from build123d import *

# Parameters (mm, degrees)
SKETCH_1_R      = 1
EXTRUDE_1_DEPTH = 1


with BuildPart() as part:
    # 草图1 → 凸台-拉伸1 (new body)
    with BuildSketch(Plane.XY):
        with BuildLine():
            Line((-1.5, 0), (-1.5, 16))
            ThreePointArc((-1.5, 16), (0, 17.5), (1.5, 16))
            Line((1.5, 16), (1.5, 0))
            ThreePointArc((1.5, 0), (0, -1.5), (-1.5, 0))
        make_face()
        with Locations((0, 16)):
            Circle(SKETCH_1_R, mode=Mode.SUBTRACT)
        with Locations((0, 8)):
            Circle(SKETCH_1_R, mode=Mode.SUBTRACT)
        with Locations((0, 12)):
            Circle(SKETCH_1_R, mode=Mode.SUBTRACT)
        Circle(SKETCH_1_R, mode=Mode.SUBTRACT)
        with Locations((0, 4)):
            Circle(SKETCH_1_R, mode=Mode.SUBTRACT)
    extrude(amount=EXTRUDE_1_DEPTH)


solid = part.part
The listing builds one solid part. Answer for the finished solid, in the listing's coordinates (mm). Round coordinates to 2 decimals unless told otherwise and drop trailing zeros. Loops run counter-clockwise (first coordinate to the right, second up) from the corner with the lowest first, then second, coordinate; pieces in that order, holes last. Notation, with made-up numbers: M -9.5,2.5 L 40.5,2.5 A16 ccw 40.5,19.5 Z; hole C 44.25,31.5 d4. An arc over 180 degrees is marked long. Return JSON: item names as keys, results as strings.
Q1. The mould has two halves that part along X. Classify faces 1 (the face through (-0.13, 4.99, 0.49)), 2 (the face through (1.5, 8.1, 0.5)), 3 (the face through (0, 17.5, 0.5)), 4 (the face through (-1.3, 8.1, 1)): released by +X, released by -X, zero draft, split by the parting line, or undercut.
Results list:
{"face 1": "undercut", "face 2": "released by +X", "face 3": "split by the parting line", "face 4": "zero draft"}
Q2. Find section B-B, the plane z = 0.3. Determine the outline of the cut face in (x, y).
Results list:
{"outline": "M -1.5,0 A1.5 ccw 1.5,0 L 1.5,16 A1.5 ccw -1.5,16 Z; hole C 0,0 d2; hole C 0,4 d2; hole C 0,8 d2; hole C 0,12 d2; hole C 0,16 d2"}
Q3. Find section A-A, the plane y = 8. Determine the outline of the cut face in (x, z).
Results list:
{"outline": "M -1.5,0 L -1,0 L -1,1 L -1.5,1 Z; M 1,0 L 1.5,0 L 1.5,1 L 1,1 Z"}
Q4. Find the intervals of material crossed by line 1 along Y through (x, z) = (0, 0.45); line 2 along X through (y, z) = (12.75, 0.1); line 3 along X through (y, z) = (11.5, 0.45), in increasing order. Write a range as from..to.
Results list:
{"line 1": "y = -1.5..-1, 1..3, 5..7, 9..11, 13..15, 17..17.5", "line 2": "x = -1.5..-0.66, 0.66..1.5", "line 3": "x = -1.5..-0.87, 0.87..1.5"}
Q5. Find section D-D, the plane y = 12.25. Determine the outline of the cut face in (x, z), plus the area to 3 significant figures.
Results list:
{"outline": "M -1.5,0 L -0.97,0 L -0.97,1 L -1.5,1 Z; M 0.97,0 L 1.5,0 L 1.5,1 L 0.97,1 Z", "area": "1.06 mm2"}
Q6. Find section C-C, the plane x = 0. Determine the outline of the cut face in (y, z), plus the area to 3 significant figures.
Results list:
{"outline": "M -1.5,0 L -1,0 L -1,1 L -1.5,1 Z; M 1,0 L 3,0 L 3,1 L 1,1 Z; M 5,0 L 7,0 L 7,1 L 5,1 Z; M 9,0 L 11,0 L 11,1 L 9,1 Z; M 13,0 L 15,0 L 15,1 L 13,1 Z; M 17,0 L 17.5,0 L 17.5,1 L 17,1 Z", "area": "9.00 mm2"}
